```python
from build123d import *

# Parameters (mm, degrees)
SKETCH1_W           = 32
SKETCH1_H           = 9.6
BOSS_EXTRUDE3_DEPTH = 8
SKETCH2_R           = 2.4
CUT_EXTRUDE6_DEPTH  = 7.8
SKETCH3_R           = 3.05
CUT_EXTRUDE7_DEPTH  = 0.8
SKETCH4_R           = 3.05
CUT_EXTRUDE8_DEPTH  = 0.8
SKETCH5_R           = 2.45
BOSS_EXTRUDE4_DEPTH = 1.8
SKETCH6_W           = 29
SKETCH6_H           = 5
CUT_EXTRUDE9_DEPTH  = 3
SKETCH7_R           = 1.5
BOSS_EXTRUDE5_DEPTH = 3


with BuildPart() as part:
    # Sketch1 → Boss-Extrude3 (new body)
    with BuildSketch(Plane(origin=(0, 0, 0), x_dir=(1, 0, 0), z_dir=(0, 1, 0))):
        with Locations((0, -1.1)):
            Rectangle(SKETCH1_W, SKETCH1_H)
    extrude(amount=BOSS_EXTRUDE3_DEPTH)

    # Sketch2 → Cut-Extrude6 (cut)
    with BuildSketch(Plane(origin=(0, 8, 0), x_dir=(1, 0, 0), z_dir=(0, 1, 0))):
        Circle(SKETCH2_R)
        with Locations((8, 0)):
            Circle(SKETCH2_R)
        with Locations((-8, 0)):
            Circle(SKETCH2_R)
    extrude(amount=-CUT_EXTRUDE6_DEPTH, mode=Mode.SUBTRACT)

    # Sketch3 → Cut-Extrude7 (cut)
    with BuildSketch(Plane(origin=(0, 8, 0), x_dir=(1, 0, 0), z_dir=(0, 1, 0))):
        Circle(SKETCH3_R)
        with Locations((8, 0)):
            Circle(SKETCH3_R)
        with Locations((-8, 0)):
            Circle(SKETCH3_R)
    extrude(amount=-CUT_EXTRUDE7_DEPTH, mode=Mode.SUBTRACT)

    # Sketch4 → Cut-Extrude8 (cut)
    with BuildSketch(Plane.XZ):
        Circle(SKETCH4_R)
        with Locations((8, 0)):
            Circle(SKETCH4_R)
        with Locations((-8, 0)):
            Circle(SKETCH4_R)
    extrude(amount=-CUT_EXTRUDE8_DEPTH, mode=Mode.SUBTRACT)

    # Sketch5 → Boss-Extrude4 (add)
    with BuildSketch(Plane(origin=(0, 0, -3.7), x_dir=(-1, 0, 0), z_dir=(0, 0, -1))):
        with Locations((-12, 4)):
            Circle(SKETCH5_R)
        with Locations((-4, 4)):
            Circle(SKETCH5_R)
        with Locations((4, 4)):
            Circle(SKETCH5_R)
        with Locations((12, 4)):
            Circle(SKETCH5_R)
    extrude(amount=BOSS_EXTRUDE4_DEPTH)

    # Sketch6 → Cut-Extrude9 (cut)
    with BuildSketch(Plane.XY.offset(5.9)):
        with Locations((0, 4)):
            Rectangle(SKETCH6_W, SKETCH6_H)
    extrude(amount=-CUT_EXTRUDE9_DEPTH, mode=Mode.SUBTRACT)

    # Sketch7 → Boss-Extrude5 (add)
    with BuildSketch(Plane.XY.offset(2.9)):
        with Locations((-8, 4)):
            Circle(SKETCH7_R)
        with Locations((0, 4)):
            Circle(SKETCH7_R)
        with Locations((8, 4)):
            Circle(SKETCH7_R)
    extrude(amount=BOSS_EXTRUDE5_DEPTH)


solid = part.part
```
Input: part model. Units: mm. Frame: model coordinates. A direction names the side the tool comes from. Give positions to 0.01 mm unless a question says otherwise; leave off trailing zeros. Write each loop counter-clockwise with the first axis right and the second up, starting at its lowest first coordinate (ties: lowest second). Pieces come first, ordered by that corner, then holes. Notation, with made-up numbers: (20, 57) - (31, 57) arc R36 cw to (31, 91) - close; hole circle Ø3 at (-2, -36). An arc over 180 degrees is marked (long way). Write item = value, one per line. Start each with the question number.
1. Section query A-A, the plane x = -12. Output: boundary loops of the cut face in (y, z).
2. Ray query, L1, parallel to X at y = 7.6, z = 0; L2, parallel to X at y = 4, z = -0.75; L3, parallel to Z at x = 0, y = 0.5. Return the intervals inside material, ascending.
3. Section query B-B, the plane x = 8. Output: boundary loops of the cut face in (y, z).
4. Mould query, pull axis Y, two halves, no side actions, for faces 6 (the flat face through (-2, 0.8, -2)), 7 (the flat face through (14.5, 4, 4)), 8 (the cylindrical face through (4.953, 7.606, -0.134)), 9 (the cylindrical face through (-9.552, 4.108, -4.587)). Classes: released by +Y, released by -Y, zero draft, split by the parting line, or undercut.
5. Section query C-C, the plane z = 0. Count the separate pieces of the cut face and the enclosed holes in it, then the cut area to 3 significant figures.
6. First-contact query: pin 1 Ø3 at (x, z) = (0.5, 0.5) entering from +Y; pin 2 Ø1.8 at (x, z) = (-7, -1.5) entering from +Y; pin 3 Ø5.5 at (x, z) = (8, 0) entering from -Y; pin 4 Ø1.5 at (x, y) = (0.5, 7) entering from -Z. Flat tips, straight axial feed; report the tip coordinate or a pass-through.
7. Access query for faces 1 (the cylindrical face through (14.448, 4.108, -4.587)), 2 (the flat face through (-10, 7.2, 2)), 3 (the cylindrical face through (-11.047, 0.394, 0.134)), 4 (the flat face through (8, 4, 5.9)), 5 (the flat face through (0, 1.5, 4)). Directions: +Z, -Z, +X, -X, +Y, -Y. A direction counts if a zero-diameter tool reaches every point of the face in a straight line with its end or side. Return the directions, or none.
Check sheet entries:
q1.outline = (0, -3.7) - (1.55, -3.7) - (1.55, -5.5) - (6.45, -5.5) - (6.45, -3.7) - (8, -3.7) - (8, 5.9) - (6.5, 5.9) - (6.5, 2.9) - (1.5, 2.9) - (1.5, 5.9) - (0, 5.9) - close
q2.L1 = -16 to -11.05, -4.95 to -3.05, 3.05 to 4.95, 11.05 to 16
q2.L2 = -16 to -10.28, -5.72 to -2.28, 2.28 to 5.72, 10.28 to 16
q2.L3 = -3.7 to -3.05, 3.05 to 5.9
q3.outline = (0, -3.7) - (8, -3.7) - (8, -3.05) - (7.2, -3.05) - (7.2, -2.4) - (0.8, -2.4) - (0.8, -3.05) - (0, -3.05) - close; (0, 3.05) - (0.8, 3.05) - (0.8, 2.4) - (7.2, 2.4) - (7.2, 3.05) - (8, 3.05) - (8, 5.9) - (6.5, 5.9) - (6.5, 2.9) - (5.5, 2.9) - (5.5, 5.9) - (2.5, 5.9) - (2.5, 2.9) - (1.5, 2.9) - (1.5, 5.9) - (0, 5.9) - close
q4.face_6 = released by -Y
q4.face_7 = undercut
q4.face_8 = zero draft
q4.face_9 = split by the parting line
q5.separate_pieces = 4
q5.enclosed_holes = 0
q5.area = 135 mm2
q6.pin_1 = through
q6.pin_2 = 7.2
q6.pin_3 = 0.8
q6.pin_4 = -3.7
q7.face_1 = -Z
q7.face_2 = +Y
q7.face_3 = -Y
q7.face_4 = +Z, +X, -X, +Y, -Y
q7.face_5 = +Z
